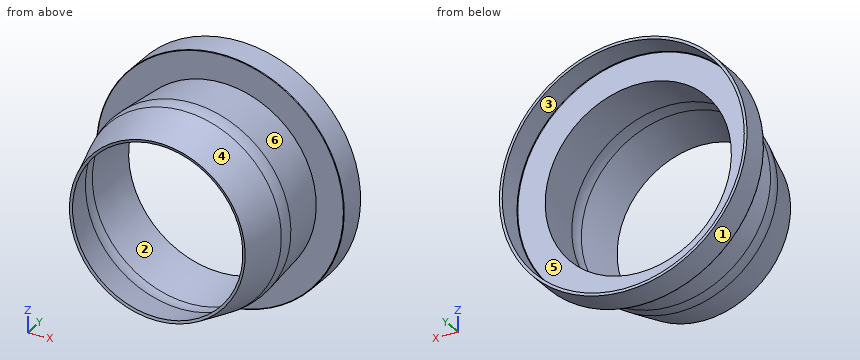
from build123d import *


with BuildPart() as part:
    # Çizim1 → Döndür1 (revolve)
    with BuildSketch(Plane.XY, mode=Mode.PRIVATE) as d_nd_r1_sk:
        with BuildLine():
            Line((-44.5, 30.888888889), (-44.5, 20.588888889))
            ThreePointArc((-44.5, 20.588888889), (-44.441421356, 20.447467533), (-44.3, 20.388888889))
            Line((-44.3, 20.388888889), (-34.545654251, 20.388888889))
            Line((-34.545654251, 20.388888889), (-36.200013267, 1.479478808))
            ThreePointArc((-36.200013267, 1.479478808), (-36.200013267, -1.135193474), (-35.74598019, -3.710143009))
            Line((-35.74598019, -3.710143009), (-31.584628047, -19.240520634))
            Line((-31.584628047, -19.240520634), (-30.618702221, -18.981701589))
            Line((-30.618702221, -18.981701589), (-34.734417582, -3.621642749))
            ThreePointArc((-34.734417582, -3.621642749), (-35.188450659, -1.046693214), (-35.188450659, 1.567979069))
            Line((-35.188450659, 1.567979069), (-33.454345749, 21.388888889))
            Line((-33.454345749, 21.388888889), (-43.3, 21.388888889))
            ThreePointArc((-43.3, 21.388888889), (-43.441421356, 21.447467533), (-43.5, 21.588888889))
            Line((-43.5, 21.588888889), (-43.5, 30.888888889))
            Line((-43.5, 30.888888889), (-44.5, 30.888888889))
        make_face()
    revolve(d_nd_r1_sk.sketch.rotate(Axis((0, 0, 0), (0, 1, 0)), 270), axis=Axis((0, 0, 0), (0, 1, 0)))


solid = part.part
Verification items for the finished model (mm, model axes). Face numbers are marked on the shaded views. A direction names the side the tool comes from. Give positions to 0.01 mm unless a question says otherwise; leave off trailing zeros. Loops run counter-clockwise (first coordinate to the right, second up) from the corner with the lowest first, then second, coordinate; pieces in that order, holes last.
1. Go/stop test with flat-tipped pins: P1, Ø6, axis at x = -34.5, y = -5, coming from the +Z side; P2, Ø1, axis at y = 14.5, z = 26, coming from the -X side; P3, Ø8, axis at y = -6, z = 15, coming from the +X side. Record where each tip stops, or that it passes through.
Derived:
P1: stops at z = 16.41
P2: stops at x = -24.07
P3: stops at x = 33.77
2. Release check for a two-part mould opening along Y. For the marked faces 3, 4, 5 and 6 record: +Y half, -Y half, draft (parallel to the pull), parting line (faces both ways), or undercut.
Derived:
face 3: draft
face 4: -Y half
face 5: +Y half
face 6: undercut
3. Cross-section at A-A on z = 0. Record the cut outline in (x, y).
Derived:
outline: (-44.5, 20.59) arc R0.2 ccw to (-44.3, 20.39) - (-34.55, 20.39) - (-36.2, 1.48) arc R15 ccw to (-35.75, -3.71) - (-31.58, -19.24) - (-30.62, -18.98) - (-34.73, -3.62) arc R15 cw to (-35.19, 1.57) - (-33.45, 21.39) - (-43.3, 21.39) arc R0.2 cw to (-43.5, 21.59) - (-43.5, 30.89) - (-44.5, 30.89) - close; (30.62, -18.98) - (31.58, -19.24) - (35.75, -3.71) arc R15 ccw to (36.2, 1.48) - (34.55, 20.39) - (44.3, 20.39) arc R0.2 ccw to (44.5, 20.59) - (44.5, 30.89) - (43.5, 30.89) - (43.5, 21.59) arc R0.2 cw to (43.3, 21.39) - (33.45, 21.39) - (35.19, 1.57) arc R15 cw to (34.73, -3.62) - close
4. Tool access check on the marked faces 1 and 2. Record the directions out of +Z, -Z, +X, -X, +Y, -Y that give a thin tool (end or side, any length) a straight path to the whole face; none if there is none.
Derived:
face 1: +Y, -Y
face 2: none
5. Cross-section at D-D on y = 16.5. Record the cut outline in (x, z), and give its area (3 significant figures).
Derived:
outline: circle Ø69.77 at (0, 0); hole circle Ø67.76 at (0, 0)
area: 217 mm2
6. Cross-section at B-B on y = 26.5. Record the cut outline in (x, z), and give its area (3 significant figures).
Derived:
outline: circle Ø89 at (0, 0); hole circle Ø87 at (0, 0)
area: 276 mm2
7. Cross-section at C-C on x = 0. Record the cut outline in (y, z), and give its area (3 significant figures).
Derived:
outline: (-19.24, -31.58) - (-3.71, -35.75) arc R15 ccw to (1.48, -36.2) - (20.39, -34.55) - (20.39, -44.3) arc R0.2 ccw to (20.59, -44.5) - (30.89, -44.5) - (30.89, -43.5) - (21.59, -43.5) arc R0.2 cw to (21.39, -43.3) - (21.39, -33.45) - (1.57, -35.19) arc R15 cw to (-3.62, -34.73) - (-18.98, -30.62) - close; (-19.24, 31.58) - (-18.98, 30.62) - (-3.62, 34.73) arc R15 cw to (1.57, 35.19) - (21.39, 33.45) - (21.39, 43.3) arc R0.2 cw to (21.59, 43.5) - (30.89, 43.5) - (30.89, 44.5) - (20.59, 44.5) arc R0.2 ccw to (20.39, 44.3) - (20.39, 34.55) - (1.48, 36.2) arc R15 ccw to (-3.71, 35.75) - close
area: 121 mm2
8. Material ranges on probe 1 along X at (y, z) = (25.75, 0); probe 2 along Y at (x, z) = (-38, 15); probe 3 along X at (y, z) = (2, 5), recorded low to high.
Derived:
probe 1: x = -44.5 to -43.5, 43.5 to 44.5
probe 2: y = 20.39 to 21.39
probe 3: x = -35.81 to -34.79, 34.79 to 35.81
